```python
from build123d import *

# Parameters (mm, degrees)
SKETCH1_W            = 160
SKETCH1_H            = 120
BOSS_EXTRUDE1_DEPTH  = 3
SKETCH2_W            = 61.9
SKETCH2_H            = 26
CUT_EXTRUDE1_DEPTH   = 10
M5_CLEARANCE_HOLE1_D = 5.5


with BuildPart() as part:
    # Sketch1 → Boss-Extrude1 (new body)
    with BuildSketch(Plane.XY):
        with Locations((80, 60)):
            Rectangle(SKETCH1_W, SKETCH1_H)
    extrude(amount=BOSS_EXTRUDE1_DEPTH)

    # Sketch2 → Cut-Extrude1 (cut)
    with BuildSketch(Plane.XY.offset(3)):
        Polygon((81.9, 26), (81.9, 0), (102, 0), (102, 45), (81.9, 45), align=None)
        with Locations((50.95, 13)):
            Rectangle(SKETCH2_W, SKETCH2_H)
    extrude(amount=-CUT_EXTRUDE1_DEPTH, mode=Mode.SUBTRACT)

    # M5 Clearance Hole1 (through all)
    with Locations(Plane.XY.offset(3)):
        with Locations((5, 114.23), (155, 5), (155, 114.23), (80, 114.23), (5, 59.615), (5, 18)):
            Hole(M5_CLEARANCE_HOLE1_D / 2)


solid = part.part
```
Can you work these out from the model? Positions are in its coordinate system, mm. Round coordinates to 2 decimals unless told otherwise and drop trailing zeros. Loops run counter-clockwise (first coordinate to the right, second up) from the corner with the lowest first, then second, coordinate; pieces in that order, holes last. Notation, with made-up numbers: M 37,80 L 79,80 A15 ccw 79,105 Z; hole C 63.25,45.25 d8. An arc over 180 degrees is marked long. Write item = value, one per line. Start each with the question number.
(1) I need wall thicknesses on line 1 along Y through (x, z) = (5, 1.1) (3 decimals); line 2 along X through (y, z) = (59.5, 0.9); line 3 along X through (y, z) = (41, 1.2). Which ranges of each line are inside material? Lowest first, please.
(2) Suppose I cut it at B-B on x = 5. Write out the boundary of the cut face in (y, z) (3 decimals).
(3) I'm going to push a flat-ended pin straight in: P1, Ø6.5, axis at x = 155, y = 114.23, coming from the +Z side. Where does the tip first touch, or does it pass through?
(4) Suppose I cut it at D-D on z = 1.4. Write out the boundary of the cut face in (x, y) (3 decimals).
(5) Suppose I cut it at C-C on y = 18. Write out the boundary of the cut face in (x, z).
(6) Suppose I cut it at A-A on x = 80. Write out the boundary of the cut face in (y, z), plus the area to 4 significant figures.
(7) If we mould it in two halves opening along X, with no side actions, what happens to faces 1 (the face through (152.38, 5.83, 1.48)), 2 (the face through (79, 61, 3))? For each: released by +X, released by -X, zero draft, split by the parting line, or undercut.
Answer block:
q1.line_1 = 0 to 15.25, 20.75 to 56.865, 62.365 to 111.48, 116.98 to 120
q1.line_2 = 0 to 2.25, 7.75 to 160
q1.line_3 = 0 to 81.9, 102 to 160
q2.outline = M 0,0 L 15.25,0 L 15.25,3 L 0,3 Z; M 20.75,0 L 56.865,0 L 56.865,3 L 20.75,3 Z; M 62.365,0 L 111.48,0 L 111.48,3 L 62.365,3 Z; M 116.98,0 L 120,0 L 120,3 L 116.98,3 Z
q3.P1 = 3
q4.outline = M 0,0 L 20,0 L 20,26 L 81.9,26 L 81.9,45 L 102,45 L 102,0 L 160,0 L 160,120 L 0,120 Z; hole C 5,18 d5.5; hole C 5,59.615 d5.5; hole C 5,114.23 d5.5; hole C 80,114.23 d5.5; hole C 155,5 d5.5; hole C 155,114.23 d5.5
q5.outline = M 0,0 L 2.25,0 L 2.25,3 L 0,3 Z; M 7.75,0 L 20,0 L 20,3 L 7.75,3 Z; M 102,0 L 160,0 L 160,3 L 102,3 Z
q6.outline = M 26,0 L 111.48,0 L 111.48,3 L 26,3 Z; M 116.98,0 L 120,0 L 120,3 L 116.98,3 Z
q6.area = 265.5 mm²
q7.face_1 = undercut
q7.face_2 = zero draft
